from build123d import *

# Parameters (mm, degrees)
SKETCH2_W          = 159.574581504
SKETCH2_H          = 68.426848692
BASE_FLANGE1_DEPTH = 3
EDGE_FLANGE1_DEPTH = 68.426848692


# Sheet-metal steps are written as plain solids
with BuildPart() as part:
    # Sketch2 → Base-Flange1 (new body)
    with BuildSketch(Plane.XY):
        Rectangle(SKETCH2_W, SKETCH2_H)
    extrude(amount=-BASE_FLANGE1_DEPTH)

    # Edge-Flange1 section (across the edge) → Edge-Flange1 (add)
    with BuildSketch(Plane(origin=(80.523890752, -34.213424346, 0), x_dir=(-1, 0, 0), z_dir=(0, 1, 0))):
        with BuildLine():
            Line((-3, 0.7366), (-3, 88))
            Line((-3, 88), (0, 88))
            Line((0, 88), (0, 0.7366))
            ThreePointArc((0, 0.7366), (0.215745145, 0.215745145), (0.7366, 0))
            Line((0.7366, 0), (0.7366, -3))
            ThreePointArc((0.7366, -3), (-1.905575199, -1.905575199), (-3, 0.7366))
        make_face()
    extrude(amount=EDGE_FLANGE1_DEPTH)


solid = part.part
The listing builds one solid part. Answer for the finished solid, in the listing's coordinates (mm). A direction names the side the tool comes from. Coordinates: 2 decimals unless noted, no trailing zeros. Loops run counter-clockwise (first coordinate to the right, second up) from the corner with the lowest first, then second, coordinate; pieces in that order, holes last.
1) Flat-ended cylindrical pins translate along their axes: pin 1 Ø1 at (y, z) = (6, 6.5) entering from -X; pin 2 Ø20.5 at (x, y) = (-16, 2) entering from +Z. Find the tip coordinate at first contact, or state that the pin passes through.
2) Find section A-A on y = 11. Write down the section's boundary in (x, z).
3) Find section B-B on x = 19. Write down the section's boundary in (y, z).
4) Find the intervals of material crossed by L1, parallel to Z at x = 52, y = 7.5; L2, parallel to X at y = -18, z = 38.5, in increasing order.
5) Find section C-C on z = 8.5. Write down the section's boundary in (x, y).
6) A tool of negligible diameter and unlimited length cuts with its end or side. For faces 1 (the face through (82.4, -0.479, -1.934)), 2 (the face through (80.524, 0, 45)), from which of +Z, -Z, +X, -X, +Y, -Y can it reach the whole face along a straight path? Write none if from no direction.
Values:
1. pin 1: stops at x = 80.52
1. pin 2: stops at z = 0
2. outline: (-79.79, -3) - (79.79, -3) arc R3.74 ccw to (83.52, 0.74) - (83.52, 88) - (80.52, 88) - (80.52, 0.74) arc R0.74 cw to (79.79, 0) - (-79.79, 0) - close
3. outline: (-34.21, -3) - (34.21, -3) - (34.21, 0) - (-34.21, 0) - close
4. L1: z = -3 to 0
4. L2: x = 80.52 to 83.52
5. outline: (80.52, -34.21) - (83.52, -34.21) - (83.52, 34.21) - (80.52, 34.21) - close
6. face 1: -Z, +X, +Y, -Y
6. face 2: +Z, -X, +Y, -Y
